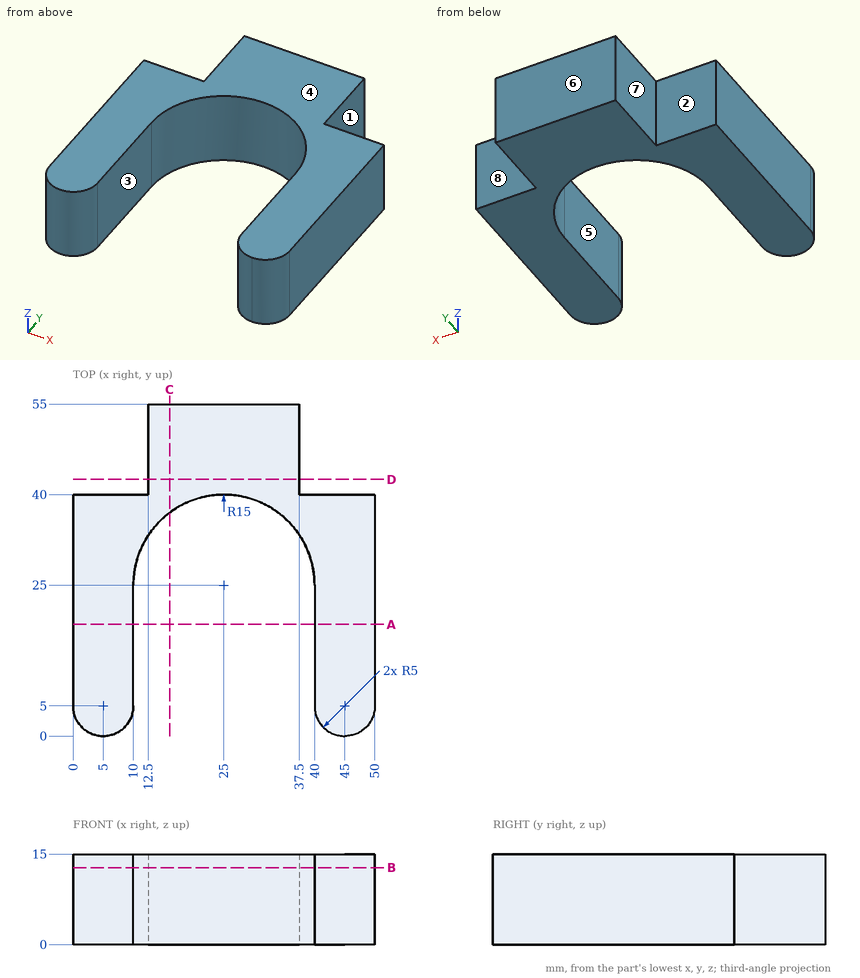
Job drawing, mm, ordinate dimensions from the low corner. One solid piece. A direction names the side the tool comes from. Round coordinates to 2 decimals unless told otherwise and drop trailing zeros. Order: outer loops, then holes, each group sorted by start corner. A loop starts at its lowest first (then second) coordinate and runs counter-clockwise, first axis right, second up. Notation, with made-up numbers: (32.5, -16.5) -> (48.5, -16.5) arc R22 cw to (48.5, 17.5) -> close; hole circle Ø7 at (68.25, -17). An arc over 180 degrees is marked (long way). Answer in a Markdown table with one row per item.
1) Which spindle directions (+Z, -Z, +X, -X, +Y, -Y) get a long thin tool onto all of the face, cutting with end or side? Do the marked faces 4, 5, 6, 7 and 8. Say none if no direction does.
Values:
| item | result |
|---|---|
| face 4 | +Z, +X, -X, +Y, -Y |
| face 5 | +Z, -Z, -Y |
| face 6 | +Z, -Z, +X, -X, +Y |
| face 7 | +Z, -Z, -X, +Y |
| face 8 | +Z, -Z, +X, +Y |
2) Band-saw the part on C-C on x = 16. Give the cut face in (y, z), and give its area (3 significant figures).
Values:
| item | result |
|---|---|
| outline | (37, 0) -> (55, 0) -> (55, 15) -> (37, 15) -> close |
| area | 270 mm2 |
3) Band-saw the part on A-A on y = 18.5. Give the cut face in (x, z), and give its area (3 significant figures).
Values:
| item | result |
|---|---|
| outline | (0, 0) -> (10, 0) -> (10, 15) -> (0, 15) -> close; (40, 0) -> (50, 0) -> (50, 15) -> (40, 15) -> close |
| area | 300 mm2 |
4) Band-saw the part on B-B on z = 12.75. Give the cut face in (x, y).
Values:
| item | result |
|---|---|
| outline | (0, 5) arc R5 ccw to (10, 5) -> (10, 25) arc R15 cw to (40, 25) -> (40, 5) arc R5 ccw to (50, 5) -> (50, 40) -> (37.5, 40) -> (37.5, 55) -> (12.5, 55) -> (12.5, 40) -> (0, 40) -> close |
5) Band-saw the part on D-D on y = 42.5. Give the cut face in (x, z), and give its area (3 significant figures).
Values:
| item | result |
|---|---|
| outline | (12.5, 0) -> (37.5, 0) -> (37.5, 15) -> (12.5, 15) -> close |
| area | 375 mm2 |
6) Wall check: L1, parallel to X at y = 21, z = 2; L2, parallel to X at y = 50.5, z = 9.5; L3, parallel to X at y = 29.5, z = 3. Give the ranges that are in metal, low to high.
Values:
| item | result |
|---|---|
| L1 | 0 to 10, 40 to 50 |
| L2 | 12.5 to 37.5 |
| L3 | 0 to 10.69, 39.31 to 50 |
7) Mould opens along X. For the marked faces 1, 2 and 3 say: released by +X, released by -X, zero draft, split by the parting line, or undercut.
Values:
| item | result |
|---|---|
| face 1 | released by +X |
| face 2 | zero draft |
| face 3 | undercut |
8) Pin check, flat tips, straight feed: P1, Ø3, axis at x = 43.5, z = 3, coming from the +Y side; P2, Ø4.5, axis at y = 50.5, z = 5.5, coming from the +X side; P3, Ø8, axis at x = 10.5, y = 15.5, coming from the -Z side; P4, Ø3, axis at x = 24, z = 4.5, coming from the -Y side. Stop position of each tip, or through.
Values:
| item | result |
|---|---|
| P1 | y = 40 |
| P2 | x = 37.5 |
| P3 | z = 0 |
| P4 | y = 39.79 |
